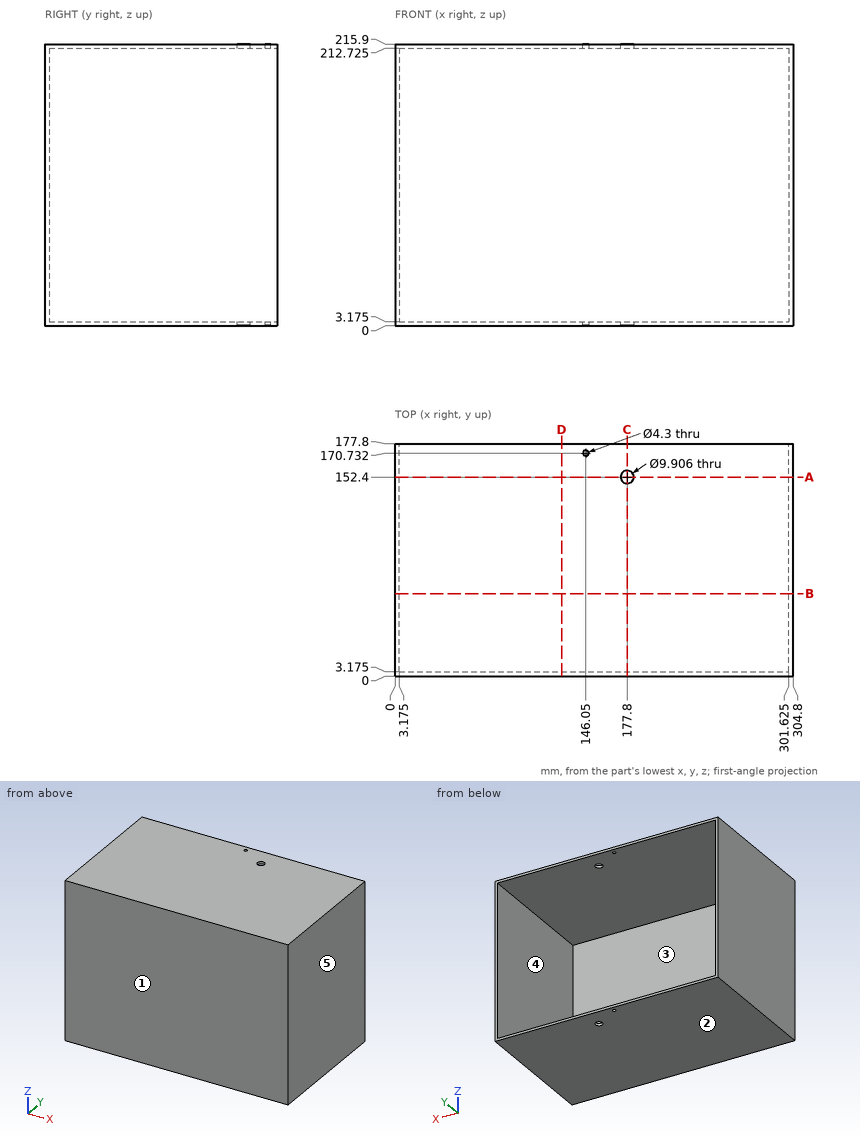
Job drawing, mm, ordinate dimensions from the low corner. One solid piece. A direction names the side the tool comes from. Round coordinates to 2 decimals unless told otherwise and drop trailing zeros. Loops run counter-clockwise (first coordinate to the right, second up) from the corner with the lowest first, then second, coordinate; pieces in that order, holes last. Notation, with made-up numbers: M 36,85.25 L 84,85.25 A20 ccw 84,121.25 Z; hole C 84,-29 d3. An arc over 180 degrees is marked long. Answer as CSV lines item,"result".
1. Cut at D-D on x = 127.5. Write the cut outline in (y, z) (3 decimals), then the cut area to 3 significant figures.
Resolved:
outline,"M 0,0 L 177.8,0 L 177.8,3.175 L 3.175,3.175 L 3.175,212.725 L 177.8,212.725 L 177.8,215.9 L 0,215.9 Z"
area,"1,790 mm²"
2. Flat gauge pin, fed straight in: P1, Ø3, axis at x = 212.5, z = 130.5, coming from the +Y side (3 decimals). Where does the tip first touch, or does it go through?
Resolved:
P1,"stops at y = 3.175"
3. Two-plate mould, pull along Z, no slides. Class the marked faces 1, 2 and 3: released by +Z, released by -Z, zero draft, split by the parting line, or undercut.
Resolved:
face 1,"zero draft"
face 2,"released by -Z"
face 3,"undercut"
4. Wall check: probe 1 along X at (y, z) = (167, 115.5) (3 decimals); probe 2 along X at (y, z) = (152, 1); probe 3 along Z at (x, y) = (40.5, 120.5) (3 decimals). Give the ranges that are in metal, low to high. Write a range as [from, to].
Resolved:
probe 1,"x = [0, 3.175], [301.625, 304.8]"
probe 2,"x = [0, 172.86], [182.74, 304.8]"
probe 3,"z = [0, 3.175], [212.725, 215.9]"
5. Cut at C-C on x = 177.8. Write the cut outline in (y, z) (3 decimals), then the cut area to 3 significant figures.
Resolved:
outline,"M 0,0 L 147.447,0 L 147.447,3.175 L 3.175,3.175 L 3.175,212.725 L 147.447,212.725 L 147.447,215.9 L 0,215.9 Z; M 157.353,0 L 177.8,0 L 177.8,3.175 L 157.353,3.175 Z; M 157.353,212.725 L 177.8,212.725 L 177.8,215.9 L 157.353,215.9 Z"
area,"1,730 mm²"
6. Cut at B-B on y = 63. Write the cut outline in (x, z) (3 decimals).
Resolved:
outline,"M 0,0 L 304.8,0 L 304.8,215.9 L 0,215.9 Z; hole M 3.175,3.175 L 301.625,3.175 L 301.625,212.725 L 3.175,212.725 Z"
7. Cut at A-A on y = 152.4. Write the cut outline in (x, z) (3 decimals), then the cut area to 3 significant figures.
Resolved:
outline,"M 0,0 L 172.847,0 L 172.847,3.175 L 3.175,3.175 L 3.175,212.725 L 172.847,212.725 L 172.847,215.9 L 0,215.9 Z; M 182.753,0 L 304.8,0 L 304.8,215.9 L 182.753,215.9 L 182.753,212.725 L 301.625,212.725 L 301.625,3.175 L 182.753,3.175 Z"
area,"3,200 mm²"
8. 3-axis set-ups, long thin cutter, end or side, ignore diameter. For the marked faces 4 and 5: which of +Z, -Z, +X, -X, +Y, -Y reach the whole face in a straight line?
Resolved:
face 4,"+Y"
face 5,"+Z, -Z, +X, +Y, -Y"
